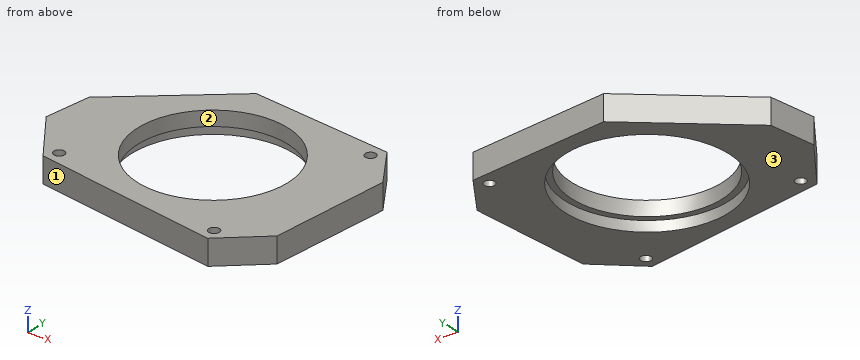
Autodesk Inventor part; units mm, degrees
ref_plane "YZ Plane" through (0, 0, 0) normal (1, 0, 0) x (0, 1, 0)
ref_plane "XZ Plane" through (0, 0, 0) normal (0, 1, 0) x (-1, 0, 0)
ref_plane "XY Plane" through (0, 0, 0) normal (0, 0, 1) x (1, 0, 0)
sketch "Sketch1" plane through (0, 0, 0) normal (0, 0, 1) x (1, 0, 0)
  line L0 (0.6045, 32.7277) -> (-43.9747, 37.2532) construction
  line L1 (-49.7733, -7.6646) -> (-5.5064, -14.6087) construction
  circle A0 centre (-43.015, 34.1404) radius 3.175 construction
  line L2 (-5.5064, -14.6087) -> (15.1919, 3.7419) construction
  line L3 (-42.0553, 31.0275) -> (-2.8152, 27.0441) construction
  line L4 (-7.3705, -8.2429) -> (-46.3358, -2.1305) construction
  line L5 (9.5291, 6.74) -> (-7.3705, -8.2429) construction
  line L6 (-2.8152, 27.0441) -> (9.7254, 8.2606) construction
  line L7 (-32.8846, 36.1274) -> (0.6045, 32.7277)
  line L8 (-32.8846, 36.1274) -> (-56.9375, 15.8971)
  line L9 (-65.2029, 14.1906) -> (-49.7733, -7.6646) construction
  line L10 (15.9639, 9.7222) -> (0.6045, 32.7277) construction
  line L11 (0.6045, 32.7277) -> (7.1877, 22.8674)
  line L12 (7.1877, 22.8674) -> (4.2625, -5.9478)
  line L13 (4.2625, -5.9478) -> (-5.5064, -14.6087)
  line L14 (-5.5064, -14.6087) -> (-49.7733, -7.6646)
  line L15 (-49.7733, -7.6646) -> (-58.6592, 4.9218)
  line L16 (-56.9375, 15.8971) -> (-58.6592, 4.9218)
  line L17 (-58.7974, 16.9461) -> (-42.0553, 31.0275) construction
  circle A1 centre (-24.6239, 11.922) radius 17.75
  circle A2 centre (-1.1053, 29.8859) radius 1.25
  circle A3 centre (-48.0546, -4.8975) radius 1.25
  circle A4 centre (-6.4384, -11.4258) radius 1.25
  point P0 (0, 0)
  dimension "d0" = 2
  dimension "d1" = 2
  dimension "d2" = 4
extrude "Extrusion1" add sketch "Sketch1" along normal blind 6
sketch "Sketch2" plane through (0, 0, 0) normal (0, 0, -1) x (-1, 0, 0)
  circle A0 centre (24.6239, 11.922) radius 17.75
  circle A1 centre (24.6239, 11.922) radius 19.25
  point P0 (0, 0)
  dimension "d5" = 38.5
extrude "Extrusion2" cut sketch "Sketch2" against normal blind 2.5
equation "\"d1\" = d0"
properties part number "TongueSideLid"
Source: CAD feature listing. Evaluate the final solid. Frame: model axes, mm. Face numbers are marked on the shaded views. Coordinates: 2 decimals unless noted, no trailing zeros. Write each loop counter-clockwise with the first axis right and the second up, starting at its lowest first coordinate (ties: lowest second). Pieces come first, ordered by that corner, then holes. Notation, with made-up numbers: M 57,-14.75 L 108,-14.75 A21 ccw 108,18.25 Z; hole C 36,48.25 d2. An arc over 180 degrees is marked long. Answer as a JSON object with one key per item and string values.
1. Contact query for flat-ended pins moving along their axis: P1, Ø2, axis at y = 12.5, z = 3.5, coming from the -X side; P2, Ø3, axis at x = -1.11, y = 29.89, coming from the -Z side; P3, Ø2, axis at x = -47, z = 2.5, coming from the +Y side; P4, Ø1, axis at x = -40.5, z = 4.5, coming from the +Y side. Output: stop coordinate, or through.
Evaluation:
{"P1": "x = -57.63", "P2": "z = 0", "P3": "y = 25.1", "P4": "y = 30.14"}
2. Cut plane B-B on x = -27. Output: boundary loops of the cut face in (y, z), plus the area to 3 significant figures.
Evaluation:
{"outline": "M -11.24,0 L -7.18,0 L -7.18,2.5 L -5.67,2.5 L -5.67,6 L -11.24,6 Z; M 29.51,2.5 L 31.02,2.5 L 31.02,0 L 35.53,0 L 35.53,6 L 29.51,6 Z", "area": "62.0 mm^2"}
3. Cut plane C-C on z = 1.15. Output: boundary loops of the cut face in (x, y).
Evaluation:
{"outline": "M -58.66,4.92 L -49.77,-7.66 L -5.51,-14.61 L 4.26,-5.95 L 7.19,22.87 L 0.6,32.73 L -32.88,36.13 L -56.94,15.9 Z; hole C -48.05,-4.9 d2.5; hole C -24.62,11.92 d38.5; hole C -6.44,-11.43 d2.5; hole C -1.11,29.89 d2.5"}
4. Draft query along X for the marked faces 1, 2 and 3. Return one class per face: released by +X, released by -X, zero draft, split by the parting line, or undercut.
Evaluation:
{"face 1": "released by -X", "face 2": "undercut", "face 3": "zero draft"}
5. Ray query, L1, parallel to Y at x = -16, z = 1.45; L2, parallel to X at y = -6, z = 3.8; L3, parallel to X at y = 4, z = 4.75. Return the intervals inside material, ascending.
Evaluation:
{"L1": "-12.96 to -5.29, 29.13 to 34.41", "L2": "-50.95 to -48.64, -47.47 to 4.2", "L3": "-58.01 to -40.51, -8.74 to 5.27"}
6. Cut plane A-A on y = 7. Output: boundary loops of the cut face in (x, z), plus the area to 3 significant figures.
Evaluation:
{"outline": "M -58.33,0 L -43.23,0 L -43.23,2.5 L -41.68,2.5 L -41.68,6 L -58.33,6 Z; M -7.57,2.5 L -6.01,2.5 L -6.01,0 L 5.58,0 L 5.58,6 L -7.57,6 Z", "area": "171 mm^2"}
